Part model, mm, in its own coordinate system. Face numbers are marked on the shaded views. A direction names the side the tool comes from. Round coordinates to 2 decimals unless told otherwise and drop trailing zeros. Order: outer loops, then holes, each group sorted by start corner. A loop starts at its lowest first (then second) coordinate and runs counter-clockwise, first axis right, second up. Notation, with made-up numbers: M -20,-10 L 16,-10 A25 cw 16,5 Z; hole C 17,33.25 d5. An arc over 180 degrees is marked long. Write each question's results on one line, items separated by ' | '. Start each with the question number.
1. Band-saw the part on B-B, the plane x = 20. List the corners of the cut face in (y, z), then the cut area to 4 significant figures.
2. Band-saw the part on C-C, the plane y = 13.5. List the corners of the cut face in (x, z).
3. Band-saw the part on A-A, the plane y = 40.5. List the corners of the cut face in (x, z), then the cut area to 3 significant figures.
4. Band-saw the part on D-D, the plane z = -11. List the corners of the cut face in (x, y), then the cut area to 3 significant figures.
5. Which spindle directions (+Z, -Z, +X, -X, +Y, -Y) get a long thin tool onto all of the face, cutting with end or side? Do the marked faces 5 and 6. Say none if no direction does.
6. Probe L1, parallel to Z at x = 30, y = 59.5; L2, parallel to X at y = 36, z = -10; L3, parallel to Y at x = 14.5, z = -7. List the from-to ranges inside material, lowest first. Write a range as [from, to].
7. Drop flat-ended pins along their axis: pin 1 Ø3.5 at (x, z) = (20, -45.25) entering from +Y; pin 2 Ø20 at (x, z) = (14, -24) entering from -Y; pin 3 Ø10 at (x, z) = (9.5, -27.5) entering from +Y. Give the stop position or say it passes through.
8. Two-plate mould, pull along Z, no slides. Class the marked faces 1, 2, 3 and 4: +Z half, -Z half, draft (parallel to the pull), parting line (faces both ways), or undercut.
```python
from build123d import *

# Parameters (mm, degrees)
SALIENTE_EXTRUIR1_DEPTH = 40
CORTAR_EXTRUIR1_DEPTH   = 79
CHAFL_N1_SIZE           = 10
CROQUIS6_R              = 2
CORTAR_EXTRUIR2_DEPTH   = 9


with BuildPart() as part:
    # Croquis1 → Saliente-Extruir1 (new body)
    with BuildSketch(Plane(origin=(0, 0, 0), x_dir=(0, 0, -1), z_dir=(1, 0, 0))):
        Polygon((0, 0), (0, 98), (3, 98), (3, 38), (52.5, 38), (52.5, 98), (55.5, 98), (55.5, 0), (52.5, 0), (52.5, 35), (3, 35), (3, 0), align=None)
    extrude(amount=SALIENTE_EXTRUIR1_DEPTH)

    # Croquis3 → Cortar-Extruir1 (cut)
    with BuildSketch(Plane.XY):
        with BuildLine():
            Line((18, 80.5), (18, 55.5))
            ThreePointArc((18, 55.5), (20, 53.5), (22, 55.5))
            Line((22, 55.5), (22, 80.5))
            ThreePointArc((22, 80.5), (20, 82.5), (18, 80.5))
        make_face()
        with BuildLine():
            Line((3, 30), (3, 5))
            ThreePointArc((3, 5), (5, 3), (7, 5))
            Line((7, 5), (7, 30))
            ThreePointArc((7, 30), (5, 32), (3, 30))
        make_face()
        with BuildLine():
            Line((33, 30), (33, 5))
            ThreePointArc((33, 5), (35, 3), (37, 5))
            Line((37, 5), (37, 30))
            ThreePointArc((37, 30), (35, 32), (33, 30))
        make_face()
    extrude(amount=-CORTAR_EXTRUIR1_DEPTH, mode=Mode.SUBTRACT)

    # Chaflán1
    chafl_n1_edges = [part.edges().sort_by_distance(p)[0] for p in [
        (0, 98, -1.5),
        (0, 98, -54),
        (40, 98, -54),
        (40, 98, -1.5),
    ]]
    chamfer(chafl_n1_edges, length=CHAFL_N1_SIZE)

    # Croquis6 → Cortar-Extruir2 (cut)
    with BuildSketch(Plane(origin=(0, 38, 0), x_dir=(1, 0, 0), z_dir=(0, 1, 0))):
        with Locations(Location((20, 45.25, 0), (0, 0, 270))):
            Circle(CROQUIS6_R)
        with Locations(Location((20, 10.25, 0), (0, 0, 270))):
            Circle(CROQUIS6_R)
    extrude(amount=-CORTAR_EXTRUIR2_DEPTH, mode=Mode.SUBTRACT)


solid = part.part
```
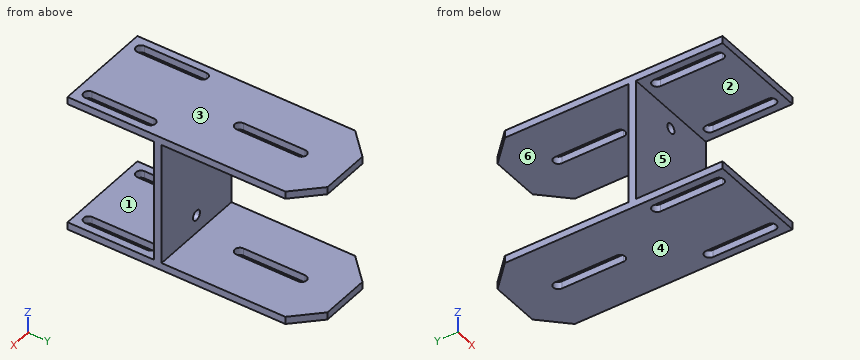
Solution:
1) outline: M 0,-55.5 L 53.5,-55.5 L 53.5,-52.5 L 38,-52.5 L 38,-47.25 L 35,-47.25 L 35,-52.5 L 0,-52.5 Z; M 0,-3 L 35,-3 L 35,-8.25 L 38,-8.25 L 38,-3 L 53.5,-3 L 53.5,0 L 0,0 Z; M 35,-43.25 L 38,-43.25 L 38,-12.25 L 35,-12.25 Z; M 82.5,-55.5 L 98,-55.5 L 98,-52.5 L 82.5,-52.5 Z; M 82.5,-3 L 98,-3 L 98,0 L 82.5,0 Z | area: 538.5 mm^2
2) outline: M 0,-55.5 L 3,-55.5 L 3,-52.5 L 0,-52.5 Z; M 0,-3 L 3,-3 L 3,0 L 0,0 Z; M 7,-55.5 L 33,-55.5 L 33,-52.5 L 7,-52.5 Z; M 7,-3 L 33,-3 L 33,0 L 7,0 Z; M 37,-55.5 L 40,-55.5 L 40,-52.5 L 37,-52.5 Z; M 37,-3 L 40,-3 L 40,0 L 37,0 Z
3) outline: M 0,-55.5 L 40,-55.5 L 40,-52.5 L 0,-52.5 Z; M 0,-3 L 40,-3 L 40,0 L 0,0 Z | area: 240 mm^2
4) outline: M 0,35 L 18.15,35 L 18.15,38 L 0,38 Z; M 21.85,35 L 40,35 L 40,38 L 21.85,38 Z | area: 109 mm^2
5) face 5: +X, -X, -Y | face 6: +X, -X, +Y
6) L1: [-55.5, -52.5], [-3, 0] | L2: [0, 18.02], [21.98, 40] | L3: [35, 38]
7) pin 1: through | pin 2: y = 35 | pin 3: y = 38
8) face 1: undercut | face 2: undercut | face 3: +Z half | face 4: -Z half
